Input: part model. Units: mm. Frame: model coordinates. Face numbers are marked on the shaded views. A direction names the side the tool comes from. Give positions to 0.01 mm unless a question says otherwise; leave off trailing zeros. Write each loop counter-clockwise with the first axis right and the second up, starting at its lowest first coordinate (ties: lowest second). Pieces come first, ordered by that corner, then holes. Notation, with made-up numbers: (2, 7.25) - (50, 7.25) arc R19 cw to (50, 28.25) - close; hole circle Ø1 at (2.25, 32). An arc over 180 degrees is marked (long way). Answer as CSV lines item,"result".
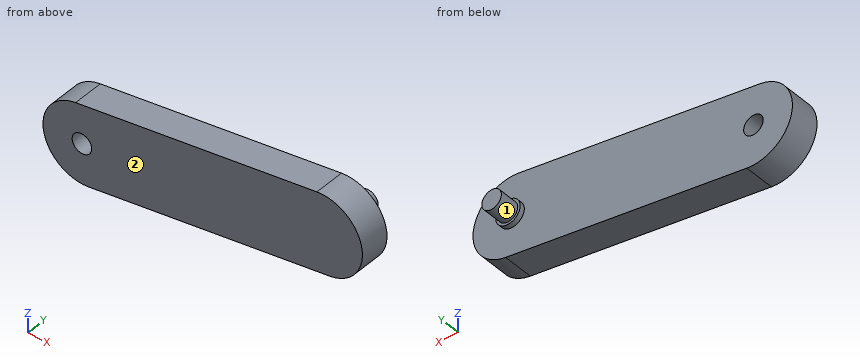
```python
from build123d import *

# Parameters (mm, degrees)
BOSS_EXTRUDE1_DEPTH   = 6
SKETCH4_R             = 2.5
BOSS_EXTRUDE3_DEPTH   = 5
BODY_MOVE_COPY1_ANGLE = 90
CUT_EXTRUDE4_START    = -4
SKETCH8_R             = 2.5
SKETCH8_R_2           = 2
CUT_EXTRUDE4_DEPTH    = 4
BODY_MOVE_COPY2_ANGLE = 180
BODY_MOVE_COPY3_ANGLE = 35
BODY_MOVE_COPY4_ANGLE = 180
SKETCH9_R             = 2
CUT_EXTRUDE5_DEPTH    = 10
BODY_MOVE_COPY5_ANGLE = 180


with BuildPart() as part:
    # Sketch1 → Boss-Extrude1 (new body)
    with BuildSketch(Plane.XY):
        with BuildLine():
            Line((0, 8), (50, 8))
            ThreePointArc((50, 8), (58, 0), (50, -8))
            Line((50, -8), (0, -8))
            ThreePointArc((0, -8), (-8, 0), (0, 8))
        make_face()
    extrude(amount=BOSS_EXTRUDE1_DEPTH)

    # Sketch4 → Boss-Extrude3 (add)
    with BuildSketch(Plane(origin=(0, 0, 0), x_dir=(-1, 0, 0), z_dir=(0, 0, -1))):
        with Locations(Location((-50, 0, 0), (0, 0, 180))):
            Circle(SKETCH4_R)
    extrude(amount=BOSS_EXTRUDE3_DEPTH)


with BuildPart() as part_1:
    # Body-Move/Copy1: moved
    add(part.part.rotate(Axis((0, 0, 11), (-1, 0, 0)), BODY_MOVE_COPY1_ANGLE))

    # Sketch8 → Cut-Extrude4 (cut)
    with BuildSketch(Plane.XZ.offset(16).offset(CUT_EXTRUDE4_START)):
        with Locations((50, 11)):
            Circle(SKETCH8_R)
        with Locations(Location((50, 11, 0), (0, 0, 270))):
            Circle(SKETCH8_R_2, mode=Mode.SUBTRACT)
    extrude(amount=CUT_EXTRUDE4_DEPTH, mode=Mode.SUBTRACT)


with BuildPart() as part_2:
    # Body-Move/Copy2: moved
    add(part_1.part.moved(Location((0, 0, 0))).rotate(Axis((-0.872729887, 0, 2.730506299), (0.9525286063620858, -4.30488929887132e-15, 0.3044490992956008)), BODY_MOVE_COPY2_ANGLE))


with BuildPart() as part_3:
    # Body-Move/Copy3: moved
    add(part_2.part.rotate(Axis((25, 0, 11), (0, 1, 0)), BODY_MOVE_COPY3_ANGLE))


with BuildPart() as part_4:
    # Body-Move/Copy4: moved
    add(part_3.part.rotate(Axis((0, 0, 11), (1, 0, 0)), BODY_MOVE_COPY4_ANGLE))

    # Sketch9 → Cut-Extrude5 (cut)
    with BuildSketch(Plane.XZ.offset(11)):
        with Locations(Location((0, 11, 0), (0, 0, 270))):
            Circle(SKETCH9_R)
    extrude(amount=-CUT_EXTRUDE5_DEPTH, mode=Mode.SUBTRACT)


with BuildPart() as part_5:
    # Body-Move/Copy5: moved
    add(part_4.part.moved(Location((0, 0, 0))).rotate(Axis((-0.706607659, -10.5, 8.976422606), (0.9969160490117142, -5.357682201744958e-14, 0.07847541795284477)), BODY_MOVE_COPY5_ANGLE))


solid = part_5.part
```
Item 1: Cut plane A-A on y = -14. Return the cut outline in (x, z).
The answers:
outline,"(-0.97, 14.79) arc R8 ccw to (1.65, -1) - (50.97, 7.21) arc R8 ccw to (48.35, 23) - close; hole circle Ø4 at (0.31, 7.09)"
Item 2: Reachability of the marked faces 1 and 2 from +Z, -Z, +X, -X, +Y, -Y: full face, straight path, thin tool, end or side. Return the list, or none.
The answers:
face 1,"+Y"
face 2,"+Z, -Z, +X, -X, -Y"
Item 3: Cut plane D-D on x = 12. Return the cut outline in (y, z), plus the area to 3 significant figures.
The answers:
outline,"(-16, 0.73) - (-10, 0.73) - (-10, 16.95) - (-16, 16.95) - close"
area,"97.3 mm²"
Item 4: Ray query, line 1 (Y direction, x = 42, z = 8); line 2 (X direction, y = -9.75, z = 15.25); line 3 (Z direction, x = 52, y = -13.5). Return the intervals inside material, ascending. Write a range as from..to.
The answers:
line 1,"-16..-10"
line 2,"47.16..52.16"
line 3,"7.46..22.76"
Item 5: Contact query for flat-ended pins moving along their axis: pin 1 (1 mm diameter, centred on x = 39, y = -11.5, fed in from -Z); pin 2 (3 mm diameter, centred on y = -6, z = 12, fed in from -X); pin 3 (5 mm diameter, centred on x = 48, y = -7, fed in from +Z). Output: stop coordinate, or through.
The answers:
pin 1,"z = 5.14"
pin 2,"x = 48.47"
pin 3,"z = 17.6"
Item 6: Cut plane C-C on y = -6. Return the cut outline in (x, z), plus the area to 3 significant figures.
The answers:
outline,"circle Ø4 at (49.66, 15.11)"
area,"12.6 mm²"
Item 7: Cut plane B-B on z = 1.75. Return the cut outline in (x, y).
The answers:
outline,"(-5.79, -16) - (18.15, -16) - (18.15, -10) - (-5.79, -10) - close"
